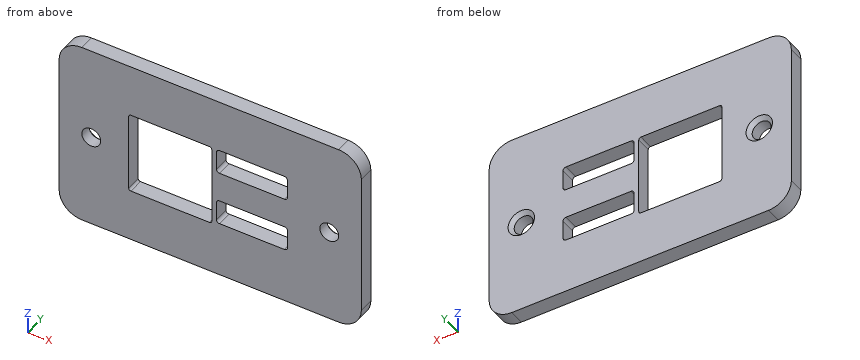
```python
from build123d import *

# Parameters (mm, degrees)
EXTRUDE_1_DEPTH            = 2
CUT_EXTRUDE_1_REACH        = 25.67
SKETCH_2_R                 = 1.25
CHAMFER_1_SIZE             = 0.5
CHAMFER_1_OF_MIRROR_3_SIZE = 0.5
CUT_EXTRUDE_2_REACH        = 25.67
CUT_EXTRUDE_3_REACH        = 25.67
CUT_EXTRUDE_4_REACH        = 25.67


with BuildPart() as part:
    # 草图1 → 凸台-拉伸1 (new body)
    with BuildSketch(Plane(origin=(0, 0, 0), x_dir=(1, 0, 0), z_dir=(0, 1, 0))):
        with BuildLine():
            Line((-17, 12.5), (17, 12.5))
            ThreePointArc((17, 12.5), (19.121320344, 11.621320344), (20, 9.5))
            Line((20, 9.5), (20, -9.5))
            ThreePointArc((20, -9.5), (19.121320344, -11.621320344), (17, -12.5))
            Line((17, -12.5), (-17, -12.5))
            ThreePointArc((-17, -12.5), (-19.121320344, -11.621320344), (-20, -9.5))
            Line((-20, -9.5), (-20, 9.5))
            ThreePointArc((-20, 9.5), (-19.121320344, 11.621320344), (-17, 12.5))
        make_face()
    extrude(amount=EXTRUDE_1_DEPTH)

    # 草图2 → 切除-拉伸1 (cut, up to next)
    with BuildSketch(Plane(origin=(0, 2, 0), x_dir=(1, 0, 0), z_dir=(0, 1, 0)), mode=Mode.PRIVATE) as cut_extrude_1_sk1:
        with Locations(Location((-15.75, 0, 0), (0, 0, 270))):
            Circle(SKETCH_2_R)
    cut_extrude_1_tool1 = extrude(cut_extrude_1_sk1.sketch, amount=-CUT_EXTRUDE_1_REACH, mode=Mode.PRIVATE) & part.part
    cut_extrude_1 = cut_extrude_1_tool1.solids().sort_by_distance((-15.75, 2, 0))[0]
    add(cut_extrude_1, mode=Mode.SUBTRACT)

    # 倒角1
    chamfer_1_edges = [part.edges().sort_by_distance(p)[0] for p in [
        (-15.75, 2, -1.25),
    ]]
    chamfer(chamfer_1_edges, length=CHAMFER_1_SIZE)

    # 镜向3: 切除-拉伸1 across plane
    add(cut_extrude_1.mirror(Plane(origin=(0, 0, 0), x_dir=(0, 0, 1), z_dir=(1, 0, 0))), mode=Mode.SUBTRACT)

    # 倒角1 of 镜向3
    chamfer_1_of_mirror_3_edges = [part.edges().sort_by_distance(p)[0] for p in [
        (15.75, 2, -1.25),
    ]]
    chamfer(chamfer_1_of_mirror_3_edges, length=CHAMFER_1_OF_MIRROR_3_SIZE)

    # 草图3 → 切除-拉伸2 (cut, up to next)
    with BuildSketch(Plane(origin=(0, 2, 0), x_dir=(1, 0, 0), z_dir=(0, 1, 0)), mode=Mode.PRIVATE) as cut_extrude_2_sk1:
        with BuildLine():
            Line((-10.5, 5.5), (-0.1, 5.5))
            ThreePointArc((-0.1, 5.5), (0.112132034, 5.412132034), (0.2, 5.2))
            Line((0.2, 5.2), (0.2, -5.2))
            ThreePointArc((0.2, -5.2), (0.112132034, -5.412132034), (-0.1, -5.5))
            Line((-0.1, -5.5), (-10.5, -5.5))
            ThreePointArc((-10.5, -5.5), (-10.712132034, -5.412132034), (-10.8, -5.2))
            Line((-10.8, -5.2), (-10.8, 5.2))
            ThreePointArc((-10.8, 5.2), (-10.712132034, 5.412132034), (-10.5, 5.5))
        make_face()
    cut_extrude_2_tool1 = extrude(cut_extrude_2_sk1.sketch, amount=-CUT_EXTRUDE_2_REACH, mode=Mode.PRIVATE) & part.part
    add(cut_extrude_2_tool1.solids().sort_by_distance((-5.3, 2, 0))[0], mode=Mode.SUBTRACT)

    # 草图4 → 切除-拉伸3 (cut, up to next)
    with BuildSketch(Plane(origin=(0, 2, 0), x_dir=(1, 0, 0), z_dir=(0, 1, 0)), mode=Mode.PRIVATE) as cut_extrude_3_sk1:
        with BuildLine():
            Line((1.22, -2.2), (9.82, -2.2))
            ThreePointArc((9.82, -2.2), (10.102842712, -2.317157288), (10.22, -2.6))
            Line((10.22, -2.6), (10.22, -5.1))
            ThreePointArc((10.22, -5.1), (10.102842712, -5.382842712), (9.82, -5.5))
            Line((9.82, -5.5), (1.22, -5.5))
            ThreePointArc((1.22, -5.5), (0.937157288, -5.382842712), (0.82, -5.1))
            Line((0.82, -5.1), (0.82, -2.6))
            ThreePointArc((0.82, -2.6), (0.937157288, -2.317157288), (1.22, -2.2))
        make_face()
    cut_extrude_3_tool1 = extrude(cut_extrude_3_sk1.sketch, amount=-CUT_EXTRUDE_3_REACH, mode=Mode.PRIVATE) & part.part
    add(cut_extrude_3_tool1.solids().sort_by_distance((5.52, 2, 3.85))[0], mode=Mode.SUBTRACT)

    # 草图5 → 切除-拉伸4 (cut, up to next)
    with BuildSketch(Plane(origin=(0, 2, 0), x_dir=(1, 0, 0), z_dir=(0, 1, 0)), mode=Mode.PRIVATE) as cut_extrude_4_sk1:
        with BuildLine():
            Line((1.22, 5.1), (9.82, 5.1))
            ThreePointArc((9.82, 5.1), (10.102842712, 4.982842712), (10.22, 4.7))
            Line((10.22, 4.7), (10.22, 2.2))
            ThreePointArc((10.22, 2.2), (10.102842712, 1.917157288), (9.82, 1.8))
            Line((9.82, 1.8), (1.22, 1.8))
            ThreePointArc((1.22, 1.8), (0.937157288, 1.917157288), (0.82, 2.2))
            Line((0.82, 2.2), (0.82, 4.7))
            ThreePointArc((0.82, 4.7), (0.937157288, 4.982842712), (1.22, 5.1))
        make_face()
    cut_extrude_4_tool1 = extrude(cut_extrude_4_sk1.sketch, amount=-CUT_EXTRUDE_4_REACH, mode=Mode.PRIVATE) & part.part
    add(cut_extrude_4_tool1.solids().sort_by_distance((5.52, 2, -3.45))[0], mode=Mode.SUBTRACT)


solid = part.part
```
The model under review builds one solid part; all positions refer to its coordinate system, in mm. Round coordinates to 2 decimals unless told otherwise and drop trailing zeros. Order: outer loops, then holes, each group sorted by start corner. A loop starts at its lowest first (then second) coordinate and runs counter-clockwise, first axis right, second up.
(1) Take a section at A-A, the plane x = -15.75. State the section outline as (y, z) points.
Working result:
outline: (0, -12.5) - (2, -12.5) - (2, -1.75) - (1.5, -1.25) - (0, -1.25) - close; (0, 1.25) - (1.5, 1.25) - (2, 1.75) - (2, 12.5) - (0, 12.5) - close
(2) Wall thickness on L1, parallel to X at y = 0.8, z = 3.5; L2, parallel to Z at x = 9, y = 1.65; L3, parallel to X at y = 1.85, z = -1: over which ranges is each line inside the solid? List them lowest first.
Working result:
L1: x = -20 to -10.8, 0.2 to 0.82, 10.22 to 20
L2: z = -12.5 to -5.1, -1.8 to 2.2, 5.5 to 12.5
L3: x = -20 to -17, -14.5 to -10.8, 0.2 to 14.5, 17 to 20
(3) Take a section at D-D, the plane z = 0. State the section outline as (x, y) points.
Working result:
outline: (-20, 0) - (-17, 0) - (-17, 1.5) - (-17.5, 2) - (-20, 2) - close; (-14.5, 0) - (-10.8, 0) - (-10.8, 2) - (-14, 2) - (-14.5, 1.5) - close; (0.2, 0) - (14.5, 0) - (14.5, 1.5) - (14, 2) - (0.2, 2) - close; (17, 0) - (20, 0) - (20, 2) - (17.5, 2) - (17, 1.5) - close
(4) For P1, Ø1.5, axis at x = -15.75, z = 0, coming from the -Y side, flat-tipped, find the tip position at first contact; note if it passes through.
Working result:
P1: passes through
(5) Take a section at B-B, the plane z = 4. State the section outline as (x, y) points, plus the area to 3 significant figures.
Working result:
outline: (-20, 0) - (-10.8, 0) - (-10.8, 2) - (-20, 2) - close; (0.2, 0) - (0.82, 0) - (0.82, 2) - (0.2, 2) - close; (10.22, 0) - (20, 0) - (20, 2) - (10.22, 2) - close
area: 39.2 mm2
(6) Take a section at C-C, the plane y = 0.55. Count the separate pieces of the cut face and the enclosed holes in it, plus the area to 3 significant figures.
Working result:
separate pieces: 1
enclosed holes: 5
area: 800 mm2
